```python
from build123d import *

# Parameters (mm, degrees)
SKETCH1_W           = 44
SKETCH1_H           = 44
BOSS_EXTRUDE1_DEPTH = 8.05
SKETCH2_W           = 39.4
SKETCH2_H           = 41.6
BOSS_EXTRUDE2_DEPTH = 8.05
SKETCH3_R           = 2
CUT_EXTRUDE1_DEPTH  = 36.031557202


with BuildPart() as part:
    # Sketch1 → Boss-Extrude1 (new body)
    with BuildSketch(Plane.XY):
        Rectangle(SKETCH1_W, SKETCH1_H)
    extrude(amount=BOSS_EXTRUDE1_DEPTH)

    # Sketch2 → Boss-Extrude2 (add)
    with BuildSketch(Plane.XY.offset(8.05)):
        Rectangle(SKETCH2_W, SKETCH2_H)
    extrude(amount=BOSS_EXTRUDE2_DEPTH)

    # Sketch3 → Cut-Extrude1 (cut, through all)
    with BuildSketch(Plane.XY.offset(16.1)):
        with Locations((-15.16, 15.25)):
            Circle(SKETCH3_R)
        with Locations((15.16, 15.25)):
            Circle(SKETCH3_R)
        with Locations((15.16, -15.25)):
            Circle(SKETCH3_R)
        with Locations((-15.16, -15.25)):
            Circle(SKETCH3_R)
    extrude(amount=-CUT_EXTRUDE1_DEPTH, mode=Mode.SUBTRACT)


solid = part.part
```
Check sheet for the modelled part. Datum: model origin and axes. Units: mm. A direction names the side the tool comes from. Give positions to 0.01 mm unless a question says otherwise; leave off trailing zeros. Write each loop counter-clockwise with the first axis right and the second up, starting at its lowest first coordinate (ties: lowest second). Pieces come first, ordered by that corner, then holes.
Item 1: Cross-section at B-B (y = -15.25). Enter the section's corners in (x, z), and give its area (3 significant figures).
Item 2: Cross-section at A-A (x = 15.16). Enter the section's corners in (y, z), and give its area (3 significant figures).
Item 3: Gauge pin test, flat ends, axial feed: pin 1 (6.5 mm diameter, centred on y = 4.5, z = 13, fed in from -X); pin 2 (4.5 mm diameter, centred on x = 15.16, y = -15.25, fed in from -Z); pin 3 (4 mm diameter, centred on x = -9, z = 11, fed in from -Y); pin 4 (6.5 mm diameter, centred on y = 4.5, z = 12.5, fed in from +X). Record the tip position at first contact, or that the pin passes through.
Item 4: Draft check along Y on faces 5 (the face through (0, 0, 0)), 6 (the face through (-15.42, -13.267, 8.163)), 7 (the face through (0, -22, 4)). Enter one of: released by +Y, released by -Y, zero draft, split by the parting line, or undercut.
Item 5: Cross-section at D-D (z = 13). Enter the section's corners in (x, y), and give its area (3 significant figures).
Item 6: Scan lines: L1, parallel to Y at x = -15.16, z = 11.25; L2, parallel to Y at x = -15.16, z = 7.25; L3, parallel to Y at x = 19, z = 15.25. Record each from-to range of solid material in increasing order.
Item 7: Access from +Z, -Z, +X, -X, +Y, -Y to the whole of each face (thin tool, end or side, straight path). Record for faces 1 (the face through (0, 20.8, 12)), 2 (the face through (-2, -21, 8.05)), 3 (the face through (-19.7, 0, 12)), 4 (the face through (19.7, 0, 12)).
Item 8: Cross-section at C-C (z = 1.75). Enter the section's corners in (x, y), and give its area (3 significant figures).
Report:
1. outline: (-22, 0) - (-17.16, 0) - (-17.16, 16.1) - (-19.7, 16.1) - (-19.7, 8.05) - (-22, 8.05) - close; (-13.16, 0) - (13.16, 0) - (13.16, 16.1) - (-13.16, 16.1) - close; (17.16, 0) - (22, 0) - (22, 8.05) - (19.7, 8.05) - (19.7, 16.1) - (17.16, 16.1) - close
1. area: 543 mm2
2. outline: (-22, 0) - (-17.25, 0) - (-17.25, 16.1) - (-20.8, 16.1) - (-20.8, 8.05) - (-22, 8.05) - close; (-13.25, 0) - (13.25, 0) - (13.25, 16.1) - (-13.25, 16.1) - close; (17.25, 0) - (22, 0) - (22, 8.05) - (20.8, 8.05) - (20.8, 16.1) - (17.25, 16.1) - close
2. area: 560 mm2
3. pin 1: stops at x = -19.7
3. pin 2: stops at z = 0
3. pin 3: stops at y = -20.8
3. pin 4: stops at x = 19.7
4. face 5: zero draft
4. face 6: undercut
4. face 7: released by -Y
5. outline: (-19.7, -20.8) - (19.7, -20.8) - (19.7, 20.8) - (-19.7, 20.8) - close; hole circle Ø4 at (-15.16, -15.25); hole circle Ø4 at (-15.16, 15.25); hole circle Ø4 at (15.16, -15.25); hole circle Ø4 at (15.16, 15.25)
5. area: 1,590 mm2
6. L1: y = -20.8 to -17.25, -13.25 to 13.25, 17.25 to 20.8
6. L2: y = -22 to -17.25, -13.25 to 13.25, 17.25 to 22
6. L3: y = -20.8 to 20.8
7. face 1: +Z, +X, -X, +Y
7. face 2: +Z
7. face 3: +Z, -X, +Y, -Y
7. face 4: +Z, +X, +Y, -Y
8. outline: (-22, -22) - (22, -22) - (22, 22) - (-22, 22) - close; hole circle Ø4 at (-15.16, -15.25); hole circle Ø4 at (-15.16, 15.25); hole circle Ø4 at (15.16, -15.25); hole circle Ø4 at (15.16, 15.25)
8. area: 1,890 mm2
